Verification items for the finished model (mm, model axes). A direction names the side the tool comes from. Coordinates: 2 decimals unless noted, no trailing zeros. Loops run counter-clockwise (first coordinate to the right, second up) from the corner with the lowest first, then second, coordinate; pieces in that order, holes last. Notation, with made-up numbers: (5.5, 68.25) -> (55.5, 68.25) arc R13 cw to (55.5, 77.25) -> close; hole circle Ø3 at (20.5, 40). An arc over 180 degrees is marked (long way). Answer as a JSON object with one key per item and string values. Group by question number.
Q1. Cross-section at D-D on x = 31. Record the boundary of the cut face in (y, z).
Q2. Set-up check for faces 5 (the flat face through (25, 16, 5)), 6 (the cylindrical face through (0.752, 18.217, 0.713)): record each of +Z, -Z, +X, -X, +Y, -Y from which the full face is reachable in a straight line by a thin tool's end or side.
Q3. Cross-section at C-C on z = 12. Record the boundary of the cut face in (x, y).
Q4. Gauge pin test, flat ends, axial feed: pin 1 Ø2 at (x, y) = (5, 16) entering from +Z; pin 2 Ø5 at (x, z) = (29.5, 8) entering from -Y; pin 3 Ø9 at (x, y) = (27, 16) entering from +Z. Record the tip position at first contact, or that the pin passes through.
Q5. Scan lines: L1, parallel to X at y = 7, z = 7.5; L2, parallel to Y at x = 45, z = 3.25; L3, parallel to Z at x = 21.5, y = 20. Record each from-to range of solid material in increasing order.
Q6. Release check for a two-part mould opening along X. For faces 1 (the flat face through (25, 36, 9)), 2 (the flat face through (9.75, 16, 10)), 3 (the flat face through (51, 18, 9)), 4 (the cylindrical face through (0.713, 35.248, 8.838)) record: released by +X, released by -X, zero draft, split by the parting line, or undercut.
Q7. Cross-section at B-B on x = 5. Record the boundary of the cut face in (y, z).
Q8. Cross-section at A-A on y = 16. Record the boundary of the cut face in (x, z), and give its area (3 significant figures).
```python
from build123d import *

# Parameters (mm, degrees)
SKETCH1_W           = 51
SKETCH1_H           = 36
BOSS_EXTRUDE1_DEPTH = 15
SKETCH2_W           = 31.5
SKETCH2_H           = 31.5
CUT_EXTRUDE1_DEPTH  = 10
SKETCH3_R           = 1.75
CUT_EXTRUDE2_DEPTH  = 65.202803677
FILLET1_R           = 0.5
FILLET2_R           = 2.5


with BuildPart() as part:
    # Sketch1 → Boss-Extrude1 (new body)
    with BuildSketch(Plane.XY):
        with Locations((25.5, 18)):
            Rectangle(SKETCH1_W, SKETCH1_H)
    extrude(amount=BOSS_EXTRUDE1_DEPTH)

    # Sketch2 → Cut-Extrude1 (cut)
    with BuildSketch(Plane.XY.offset(15)):
        with Locations((25.5, 15.75)):
            Rectangle(SKETCH2_W, SKETCH2_H)
    extrude(amount=-CUT_EXTRUDE1_DEPTH, mode=Mode.SUBTRACT)

    # Sketch3 → Cut-Extrude2 (cut, through all)
    with BuildSketch(Plane.XY.offset(15)):
        with Locations((5, 31)):
            Circle(SKETCH3_R)
        with Locations((5, 16)):
            Circle(SKETCH3_R)
        with Locations((46, 31)):
            Circle(SKETCH3_R)
        with Locations((46, 16)):
            Circle(SKETCH3_R)
    extrude(amount=-CUT_EXTRUDE2_DEPTH, mode=Mode.SUBTRACT)

    # Fillet1
    fillet1_edges = [part.edges().sort_by_distance(p)[0] for p in [
        (25.5, 0, 5),
        (41.25, 0, 10),
        (9.75, 15.75, 5),
        (9.75, 0, 10),
        (25.5, 31.5, 5),
        (9.75, 31.5, 10),
        (41.25, 15.75, 5),
        (41.25, 31.5, 10),
    ]]
    fillet(fillet1_edges, radius=FILLET1_R)

    # Fillet2
    fillet2_edges = [part.edges().sort_by_distance(p)[0] for p in [
        (25.5, 36, 0),
        (51, 18, 0),
        (25.5, 0, 0),
        (0, 18, 0),
        (0, 36, 7.5),
        (51, 36, 7.5),
        (51, 0, 7.5),
        (0, 0, 7.5),
    ]]
    fillet(fillet2_edges, radius=FILLET2_R)


solid = part.part
```
Computed values:
{
 "1": {"outline": "(0, 2.5) arc R2.5 ccw to (2.5, 0) -> (33.5, 0) arc R2.5 ccw to (36, 2.5) -> (36, 15) -> (31.5, 15) -> (31.5, 5.5) arc R0.5 cw to (31, 5) -> (0.5, 5) arc R0.5 ccw to (0, 4.5) -> close"},
 "2": {"face 5": "+Z, -Y", "face 6": "-Z, -X, +Y, -Y"},
 "3": {"outline": "(0, 2.5) arc R2.5 ccw to (2.5, 0) -> (9.25, 0) arc R0.5 ccw to (9.75, 0.5) -> (9.75, 31) arc R0.5 cw to (10.25, 31.5) -> (40.75, 31.5) arc R0.5 cw to (41.25, 31) -> (41.25, 0.5) arc R0.5 ccw to (41.75, 0) -> (48.5, 0) arc R2.5 ccw to (51, 2.5) -> (51, 33.5) arc R2.5 ccw to (48.5, 36) -> (2.5, 36) arc R2.5 ccw to (0, 33.5) -> close; hole circle Ø3.5 at (5, 16); hole circle Ø3.5 at (5, 31); hole circle Ø3.5 at (46, 16); hole circle Ø3.5 at (46, 31)"},
 "4": {"pin 1": "passes through", "pin 2": "stops at y = 31.5", "pin 3": "stops at z = 5"},
 "5": {"L1": "x = 0 to 9.75, 41.25 to 51", "L2": "y = 0 to 14.56, 17.44 to 29.56, 32.44 to 36", "L3": "z = 0 to 5"},
 "6": {"face 1": "zero draft", "face 2": "undercut", "face 3": "released by +X", "face 4": "released by -X"},
 "7": {"outline": "(0, 2.5) arc R2.5 ccw to (2.5, 0) -> (14.25, 0) -> (14.25, 15) -> (0, 15) -> close; (17.75, 0) -> (29.25, 0) -> (29.25, 15) -> (17.75, 15) -> close; (32.75, 0) -> (33.5, 0) arc R2.5 ccw to (36, 2.5) -> (36, 15) -> (32.75, 15) -> close"},
 "8": {"outline": "(0, 2.5) arc R2.5 ccw to (2.5, 0) -> (3.25, 0) -> (3.25, 15) -> (0, 15) -> close; (6.75, 0) -> (44.25, 0) -> (44.25, 15) -> (41.25, 15) -> (41.25, 5.5) arc R0.5 cw to (40.75, 5) -> (10.25, 5) arc R0.5 cw to (9.75, 5.5) -> (9.75, 15) -> (6.75, 15) -> close; (47.75, 0) -> (48.5, 0) arc R2.5 ccw to (51, 2.5) -> (51, 15) -> (47.75, 15) -> close", "area": "342 mm²"}
}
